Design review of the part shown in the three views and the two pictorial views. Dimensions are in mm from the part's minimum x, y and z. A direction names the side the tool comes from. Give positions to 0.01 mm unless a question says otherwise; leave off trailing zeros. Loops run counter-clockwise (first coordinate to the right, second up) from the corner with the lowest first, then second, coordinate; pieces in that order, holes last.
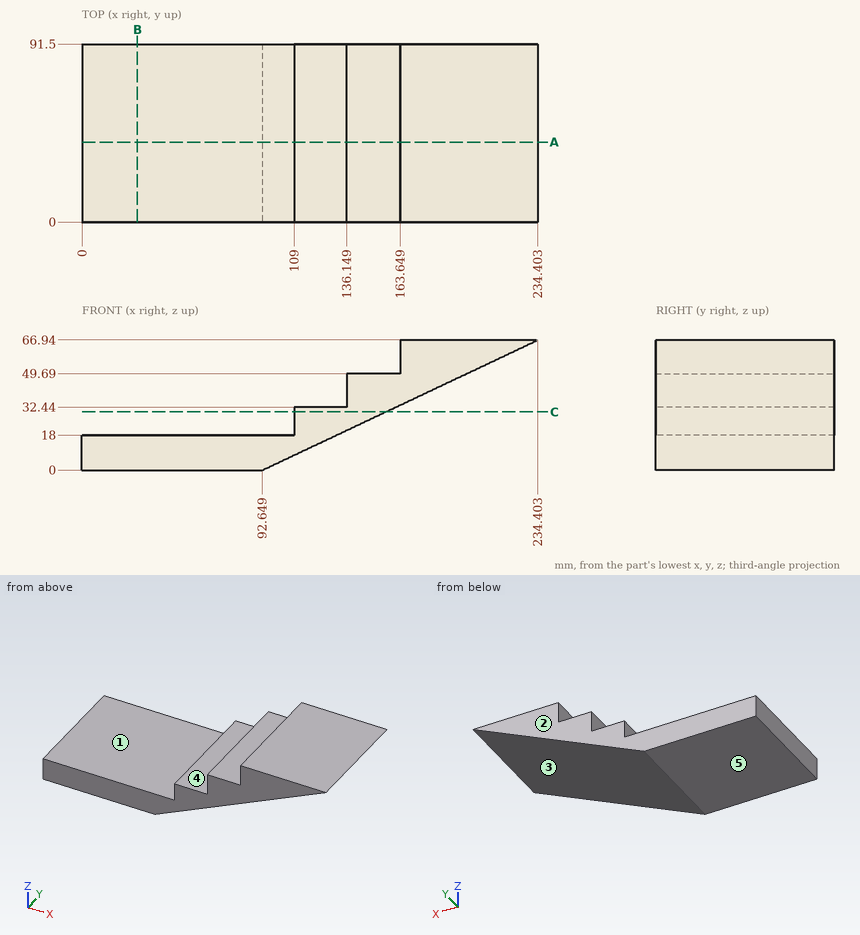
Q1. Take a section at B-B (x = 28.5). Give the boundary of the cut face in (y, z).
Results:
outline: (0, 0) - (91.5, 0) - (91.5, 18) - (0, 18) - close
Q2. Draft analysis for pull direction Z (two halves, no side actions). For the marked faces 1, 2 and 3, state which applies: pulls with the +Z half, pulls with the -Z half, needs draft (parallel to the pull), parting line crosses it, or undercut.
Results:
face 1: pulls with the +Z half
face 2: needs draft
face 3: pulls with the -Z half
Q3. Take a section at A-A (y = 41). Give the boundary of the cut face in (x, z), plus the area to 3 significant figures.
Results:
outline: (0, 0) - (92.65, 0) - (234.4, 66.94) - (163.65, 66.94) - (163.65, 49.69) - (136.15, 49.69) - (136.15, 32.44) - (109, 32.44) - (109, 18) - (0, 18) - close
area: 4,200 mm2
Q4. Take a section at C-C (z = 30). Give the boundary of the cut face in (x, y), plus the area to 3 significant figures.
Results:
outline: (109, 0) - (156.18, 0) - (156.18, 91.5) - (109, 91.5) - close
area: 4,320 mm2
Q5. Wall thickness on line 1 (Z direction, x = 33, y = 16.5); line 2 (Z direction, x = 99.5, y = 11.5) (1 decimal); line 3 (X direction, y = 76.5, z = 26.5) (1 decimal): over which ranges is each line inside the solid? List them lowest first.
Results:
line 1: z = 0 to 18
line 2: z = 3.2 to 18
line 3: x = 109 to 148.8
Q6. Insertion check: pin 1 (12 mm diameter, centred on y = 74, z = 50, fed in from -X); pin 2 (22 mm diameter, centred on x = 148.5, y = 56.5, fed in from +Z); pin 3 (5 mm diameter, centred on x = 168.5, y = 66.5, fed in from -Z); pin 4 (12 mm diameter, centred on x = 191, z = 38, fed in from +Y). Each pin has a flat end and moves straight along its axis. Give the tip position at first contact, or say it passes through.
Results:
pin 1: stops at x = 136.15
pin 2: stops at z = 49.69
pin 3: stops at z = 34.64
pin 4: passes through
Q7. Tool access review of the marked faces 4 and 5: name each direction out of +Z, -Z, +X, -X, +Y, -Y from which nothing blocks a thin tool from reaching the whole face with its end or side.
Results:
face 4: +Z, -X, +Y, -Y
face 5: -Z, +X, -X, +Y, -Y
